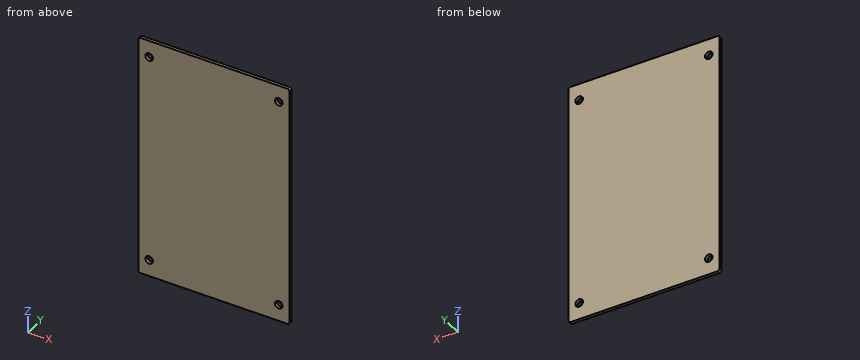
from build123d import *

# Parameters (mm, degrees)
SKETCH1_R           = 1.75
BOSS_EXTRUDE1_DEPTH = 1.5
FILLET1_R           = 7
FILLET2_R           = 1
FILLET3_R           = 50
SKETCH2_W           = 103.402572328
SKETCH2_H           = 105.78008475
CUT_EXTRUDE1_DEPTH  = 10


with BuildPart() as part:
    # Sketch1 → Boss-Extrude1 (new body)
    with BuildSketch(Plane(origin=(0, 0, 0), x_dir=(1, 0, 0), z_dir=(0, 1, 0))):
        Polygon((-35, -55), (-28, -55), (-28, -132), (0, -144), (28, -132), (28, -55), (35, -55), (35, 55), (28, 55), (28, 132), (0, 144), (-28, 132), (-28, 55), (-35, 55), align=None)
        with Locations(Location((-30, 47.5, 0), (0, 0, 270))):
            Circle(SKETCH1_R, mode=Mode.SUBTRACT)
        with Locations(Location((30, 47.5, 0), (0, 0, 270))):
            Circle(SKETCH1_R, mode=Mode.SUBTRACT)
        with Locations(Location((30, -47.5, 0), (0, 0, 270))):
            Circle(SKETCH1_R, mode=Mode.SUBTRACT)
        with Locations(Location((-30, -47.5, 0), (0, 0, 270))):
            Circle(SKETCH1_R, mode=Mode.SUBTRACT)
    extrude(amount=BOSS_EXTRUDE1_DEPTH)

    # Fillet1
    fillet1_edges = [part.edges().sort_by_distance(p)[0] for p in [
        (-28, 0.75, 55),
        (28, 0.75, 55),
        (28, 0.75, -55),
        (-28, 0.75, -55),
    ]]
    fillet(fillet1_edges, radius=FILLET1_R - 0.0001)  # a hair under: the kernel refuses the full size

    # Fillet2
    fillet2_edges = [part.edges().sort_by_distance(p)[0] for p in [
        (35, 0.75, -55),
        (35, 0.75, 55),
        (-35, 0.75, 55),
        (-35, 0.75, -55),
    ]]
    fillet(fillet2_edges, radius=FILLET2_R)

    # Fillet3
    fillet3_edges = [part.edges().sort_by_distance(p)[0] for p in [
        (0, 0.75, 144),
        (0, 0.75, -144),
    ]]
    fillet(fillet3_edges, radius=FILLET3_R)

    # Sketch2 → Cut-Extrude1 (cut)
    with BuildSketch(Plane(origin=(0, 1.5, 0), x_dir=(1, 0, 0), z_dir=(0, 1, 0))):
        with Locations((-17.576286164, 107.944945183)):
            Rectangle(SKETCH2_W, SKETCH2_H)
    cut_extrude1 = extrude(amount=-CUT_EXTRUDE1_DEPTH, mode=Mode.SUBTRACT)

    # Mirror1: Cut-Extrude1 across plane
    add(cut_extrude1.mirror(Plane.XY), mode=Mode.SUBTRACT)


solid = part.part
Geometry: final body of the model. Coordinates: model frame, mm. Coordinates: 2 decimals unless noted, no trailing zeros. Order: outer loops, then holes, each group sorted by start corner. A loop starts at its lowest first (then second) coordinate and runs counter-clockwise, first axis right, second up. Notation, with made-up numbers: (88.25, 21.25) - (121.25, 21.25) arc R30 ccw to (121.25, 59.25) - close; hole circle Ø7 at (-36, 7.5). An arc over 180 degrees is marked (long way). Use one line per item in the form item = value.
1) Ray query, L1, parallel to X at y = 1, z = 47.5; L2, parallel to Z at x = 30.5, y = 0.4. Return the intervals inside material, ascending.
Solutions:
L1 = -35 to -31.75, -28.25 to 28.25, 31.75 to 35
L2 = -55.05 to -49.18, -45.82 to 45.82, 49.18 to 55.05
2) Pin query (flat end, axial travel): pin 1 (3 mm diameter, centred on x = -30, z = 47.5, fed in from -Y). Return the tip coordinate at first contact, or that it passes through.
Solutions:
pin_1 = through
3) Section B-B (x = 30). Return loops of the section in (y, z), then the cut area to 3 significant figures.
Solutions:
outline = (0, -55.05) - (1.5, -55.05) - (1.5, -49.25) - (0, -49.25) - close; (0, -45.75) - (1.5, -45.75) - (1.5, 45.75) - (0, 45.75) - close; (0, 49.25) - (1.5, 49.25) - (1.5, 55.05) - (0, 55.05) - close
area = 155 mm^2
4) Section A-A (z = -47.5). Return loops of the section in (x, y), then the cut area to 3 significant figures.
Solutions:
outline = (-35, 0) - (-31.75, 0) - (-31.75, 1.5) - (-35, 1.5) - close; (-28.25, 0) - (28.25, 0) - (28.25, 1.5) - (-28.25, 1.5) - close; (31.75, 0) - (35, 0) - (35, 1.5) - (31.75, 1.5) - close
area = 94.5 mm^2
